The listing builds one solid part. Answer for the finished solid, in the listing's coordinates (mm). Face numbers are marked on the shaded views. Round coordinates to 2 decimals unless told otherwise and drop trailing zeros. Loops run counter-clockwise (first coordinate to the right, second up) from the corner with the lowest first, then second, coordinate; pieces in that order, holes last. Notation, with made-up numbers: (19.25, -24) - (47.25, -24) arc R18 cw to (47.25, -3) - close; hole circle Ø1 at (38.25, 82). An arc over 180 degrees is marked (long way). One line per question, with ' | ' between items. Start each with the question number.
from build123d import *

# Parameters (mm, degrees)
BOSS_EXTRUDE1_DEPTH      = 12
BOSS_EXTRUDE1_DEPTH_BACK = 18
SKETCH1_R                = 6.825
CUT_EXTRUDE1_DEPTH       = 21.424525698
CUT_EXTRUDE1_DEPTH_BACK  = 21.424525698
SKETCH2_R                = 2.6
SKETCH2_R_2              = 1.35
FILLET1_R                = 1
FILLET2_R                = 0.5


with BuildPart() as part:
    # Sketch1 → Boss-Extrude1 (new, two sides: drawn at the far end of the back side and taken through both)
    with BuildSketch(Plane.XY.offset(-BOSS_EXTRUDE1_DEPTH_BACK)):
        Circle(SKETCH1_R)
    extrude(amount=BOSS_EXTRUDE1_DEPTH + BOSS_EXTRUDE1_DEPTH_BACK)

    # Sketch2 → Cut-Extrude1 (cut, two sides: drawn at the far end of the back side and taken through both)
    with BuildSketch(Plane(origin=(0, 0, 0), x_dir=(1, 0, 0), z_dir=(0, 1, 0)).offset(-CUT_EXTRUDE1_DEPTH_BACK)):
        with Locations(Location((0, 0, 0), (0, 0, 270))):
            Circle(SKETCH2_R)
        with Locations(Location((0, 13.5, 0), (0, 0, 270))):
            Circle(SKETCH2_R_2)
    extrude(amount=CUT_EXTRUDE1_DEPTH + CUT_EXTRUDE1_DEPTH_BACK, mode=Mode.SUBTRACT)

    # Fillet1
    fillet1_edges = [part.edges().sort_by_distance(p)[0] for p in [
        (-6.825, 0, 12),
        (-6.825, 0, -18),
    ]]
    fillet(fillet1_edges, radius=FILLET1_R)

    # Fillet2
    fillet2_edges = [part.edges().sort_by_distance(p)[0] for p in [
        (1e-09, 6.825, -2.600000001),
        (0, -6.825, -2.600000002),
    ]]
    fillet(fillet2_edges, radius=FILLET2_R)


solid = part.part
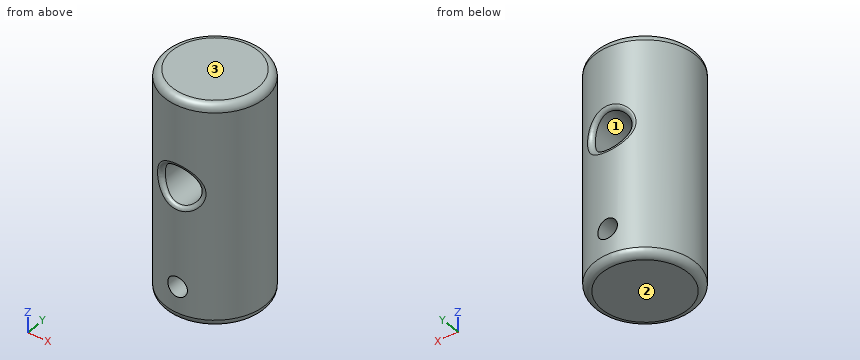
(1) Find section B-B on x = 0. Count the separate pieces of the cut face and the enclosed holes in it, plus the area to 3 significant figures.
(2) Each of these flat-tipped pins is pushed along its axis until it touches: P1, Ø1.5, axis at y = -3, z = -9, coming from the +X side; P2, Ø2, axis at x = -4.5, z = -7, coming from the +Y side; P3, Ø6, axis at x = -4.5, z = 7.5, coming from the -Y side; P4, Ø5, axis at x = 2, z = -4.5, coming from the +Y side (3 decimals). Where does it stop, or does it pass through?
(3) Find section A-A on y = 0. Write down the section's boundary in (x, z) (3 decimals).
(4) Determine the mould class of the marked faces 1, 2 and 3 for opening direction Z: pulls with the +Z half, pulls with the -Z half, needs draft (parallel to the pull), parting line crosses it, or undercut.
(5) Consider L1, parallel to Z at x = 0, y = -3.75; L2, parallel to X at y = -2.75, z = -13.5; L3, parallel to X at y = -3.5, z = 0. Determine where each line is inside the solid, lowest interval first.
(6) Find section C-C on z = -6.5. Write down the section's boundary in (x, y) (3 decimals), plus the area to 3 significant figures.
(7) Find section D-D on z = -13.5. Write down the section's boundary in (x, y) (3 decimals).
Answer below:
1) separate pieces: 3 | enclosed holes: 0 | area: 301 mm2
2) P1: x = 6.44 | P2: y = 5.86 | P3: y = -6.66 | P4: y = 6.825
3) outline: (-6.825, -17) arc R1 ccw to (-5.825, -18) - (5.825, -18) arc R1 ccw to (6.825, -17) - (6.825, 11) arc R1 ccw to (5.825, 12) - (-5.825, 12) arc R1 ccw to (-6.825, 11) - close; hole circle Ø5.2 at (0, 0); hole circle Ø2.7 at (0, -13.5)
4) face 1: undercut | face 2: pulls with the -Z half | face 3: pulls with the +Z half
5) L1: -18 to -14.85, -12.15 to -2.6, 2.6 to 12 | L2: -6.25 to -1.35, 1.35 to 6.25 | L3: -5.86 to -2.6, 2.6 to 5.86
6) outline: circle Ø13.65 at (0, 0) | area: 146 mm2
7) outline: (-1.35, -6.69) - (-1.35, 6.69) arc R6.825 ccw to start; (1.35, -6.69) arc R6.825 ccw to (1.35, 6.69) - close
